```python
from build123d import *

# Parameters (mm, degrees)
BOSS_EXTRUDE1_START       = -4
BOSS_EXTRUDE1_OUTLINE_R   = 2.2
BOSS_EXTRUDE1_OUTLINE_R_2 = 1.025
BOSS_EXTRUDE1_OUTLINE_R_3 = 6.575
BOSS_EXTRUDE1_DEPTH       = 4
SKETCH3_R                 = 8.875
SKETCH3_R_2               = 7.075
CUT_EXTRUDE1_DEPTH        = 1.05
BOSS_EXTRUDE2_START       = -4
SKETCH4_R                 = 1.025
BOSS_EXTRUDE2_DEPTH       = 0.75
FILLET1_R                 = 1
BOSS_EXTRUDE3_START       = -5
SKETCH5_R                 = 32.5
SKETCH5_R_2               = 1.025
SKETCH5_R_3               = 8.875
BOSS_EXTRUDE3_DEPTH       = 5
SKETCH6_R                 = 2.65
CUT_EXTRUDE2_DEPTH        = 5
SKETCH7_R                 = 20.6
SKETCH7_R_2               = 15.6
CUT_EXTRUDE3_DEPTH        = 2.5
BOSS_EXTRUDE4_START       = 1
SKETCH8_R                 = 1.025
BOSS_EXTRUDE4_DEPTH       = 1


# Read off the part's stored shape, not the designer's step: Boss-Extrude1
with BuildPart() as part:
    # Boss-Extrude1 outline → Boss-Extrude1 (new body)
    with BuildSketch(Plane.XY.offset(BOSS_EXTRUDE1_START)):
        with BuildLine():
            Line((-5.8, 12.8), (-5.8, -12.8))
            ThreePointArc((-5.8, -12.8), (-1.992388155, -21.992388155), (7.2, -25.8))
            Line((7.2, -25.8), (32.8, -25.8))
            ThreePointArc((32.8, -25.8), (41.992388155, -21.992388155), (45.8, -12.8))
            Line((45.8, -12.8), (45.8, 12.8))
            ThreePointArc((45.8, 12.8), (41.992388155, 21.992388155), (32.8, 25.8))
            Line((32.8, 25.8), (7.2, 25.8))
            ThreePointArc((7.2, 25.8), (-1.992388155, 21.992388155), (-5.8, 12.8))
        make_face()
        with Locations((25, -22)):
            Circle(BOSS_EXTRUDE1_OUTLINE_R, mode=Mode.SUBTRACT)
        with Locations((20, -11.1252)):
            Circle(BOSS_EXTRUDE1_OUTLINE_R_2, mode=Mode.SUBTRACT)
        with Locations((-2, 0)):
            Circle(BOSS_EXTRUDE1_OUTLINE_R, mode=Mode.SUBTRACT)
        with Locations((20, 0)):
            Circle(BOSS_EXTRUDE1_OUTLINE_R_3, mode=Mode.SUBTRACT)
        with Locations((20, 11.1252)):
            Circle(BOSS_EXTRUDE1_OUTLINE_R_2, mode=Mode.SUBTRACT)
        with Locations((42, 0)):
            Circle(BOSS_EXTRUDE1_OUTLINE_R, mode=Mode.SUBTRACT)
        with Locations((25, 22)):
            Circle(BOSS_EXTRUDE1_OUTLINE_R, mode=Mode.SUBTRACT)
    extrude(amount=BOSS_EXTRUDE1_DEPTH)

    # Sketch3 → Cut-Extrude1 (cut)
    with BuildSketch(Plane.XY):
        with Locations((20, 0)):
            Circle(SKETCH3_R)
        with Locations((20, 0)):
            Circle(SKETCH3_R_2, mode=Mode.SUBTRACT)
    extrude(amount=-CUT_EXTRUDE1_DEPTH, mode=Mode.SUBTRACT)

    # Sketch4 → Boss-Extrude2 (add)
    with BuildSketch(Plane.XY.offset(BOSS_EXTRUDE2_START)):
        with Locations((20, 11.1252)):
            Circle(SKETCH4_R)
        with Locations((20, -11.1252)):
            Circle(SKETCH4_R)
    extrude(amount=BOSS_EXTRUDE2_DEPTH)

    # Fillet1
    fillet1_edges = [part.edges().sort_by_distance(p)[0] for p in [
        (18.975, 11.1252, -3.25),
        (18.975, -11.1252, -3.25),
    ]]
    fillet(fillet1_edges, radius=FILLET1_R)

    # Sketch5 → Boss-Extrude3 (add)
    with BuildSketch(Plane.XY.offset(BOSS_EXTRUDE3_START)):
        with Locations((20, 0)):
            Circle(SKETCH5_R)
        with Locations((20, -11.1252)):
            Circle(SKETCH5_R_2, mode=Mode.SUBTRACT)
        with Locations((20, 11.1252)):
            Circle(SKETCH5_R_2, mode=Mode.SUBTRACT)
        with Locations((20, 0)):
            Circle(SKETCH5_R_3, mode=Mode.SUBTRACT)
    extrude(amount=BOSS_EXTRUDE3_DEPTH)

    # Sketch6 → Cut-Extrude2 (cut)
    with BuildSketch(Plane.XY):
        with Locations((-8.5, 0)):
            Circle(SKETCH6_R)
        with Locations((20, 28.5)):
            Circle(SKETCH6_R)
        with Locations((48.5, 0)):
            Circle(SKETCH6_R)
        with Locations((20, -28.5)):
            Circle(SKETCH6_R)
    extrude(amount=-CUT_EXTRUDE2_DEPTH, mode=Mode.SUBTRACT)

    # Sketch7 → Cut-Extrude3 (cut)
    with BuildSketch(Plane(origin=(0, 0, -5), x_dir=(-1, 0, 0), z_dir=(0, 0, -1))):
        with Locations((-20, 0)):
            Circle(SKETCH7_R)
        with Locations((-20, 0)):
            Circle(SKETCH7_R_2, mode=Mode.SUBTRACT)
    extrude(amount=-CUT_EXTRUDE3_DEPTH, mode=Mode.SUBTRACT)

    # Sketch8 → Boss-Extrude4 (add)
    with BuildSketch(Plane(origin=(0, 0, -4), x_dir=(-1, 0, 0), z_dir=(0, 0, -1)).offset(BOSS_EXTRUDE4_START)):
        with Locations(Location((-20, -11.1252, 0), (0, 0, 180))):
            Circle(SKETCH8_R)
        with Locations(Location((-20, 11.1252, 0), (0, 0, 180))):
            Circle(SKETCH8_R)
    extrude(amount=-BOSS_EXTRUDE4_DEPTH)


solid = part.part
```
Check sheet for the modelled part. Datum: model origin and axes. Units: mm. A direction names the side the tool comes from. Coordinates: 2 decimals unless noted, no trailing zeros. Order: outer loops, then holes, each group sorted by start corner. A loop starts at its lowest first (then second) coordinate and runs counter-clockwise, first axis right, second up. Notation, with made-up numbers: M 9.25,20 L 44.25,20 A32 cw 44.25,58 Z; hole C 41,48.5 d5. An arc over 180 degrees is marked long. Write each question's results on one line, items separated by ' | '. Start each with the question number.
1. Material ranges on probe 1 along Y at (x, z) = (20, -4.35) (3 decimals); probe 2 along Y at (x, z) = (20, -1.85) (3 decimals); probe 3 along X at (y, z) = (-6, -3.9), recorded low to high.
2. Cross-section at A-A on y = 28.5. Record the cut outline in (x, z).
3. Cross-section at C-C on y = 0. State how many separate pieces and enclosed holes the cut face has, and give its area (3 significant figures).
4. Mould release check, pull along X, two halves, no side actions. Record for faces 1 (the face through (36.35, -12.53, -3.77)), 2 (the face through (41, 0, -5)): +X half, -X half, draft (parallel to the pull), parting line (faces both ways), or undercut.
5. Cross-section at B-B on x = 48.5. Record the cut outline in (y, z), and give its area (3 significant figures).
6. Access from +Z, -Z, +X, -X, +Y, -Y to the whole of each face (thin tool, end or side, straight path). Record for faces 3 (the face through (5.12, 4.69, -3.77)), 4 (the face through (18.466, -6.907, -0.518)), 5 (the face through (27, 7, -5)).
7. Cross-section at D-D on x = 10. Record the cut outline in (y, z), and give its area (3 significant figures).
8. Go/stop test with flat-tipped pins: P1, Ø14, axis at x = 20, y = 0, coming from the -Z side; P2, Ø1.5, axis at y = 14.5, z = -1, coming from the -X side; P3, Ø2, axis at y = -11, z = -1, coming from the -X side. Record where each tip stops, or that it passes through.
Checks:
1) probe 1: y = -32.5 to -31.15, -25.85 to -20.6, -15.6 to -8.875, 8.875 to 15.6, 20.6 to 25.85, 31.15 to 32.5 | probe 2: y = -32.5 to -31.15, -25.85 to -12.15, -10.1 to -6.575, 6.575 to 10.1, 12.15 to 25.85, 31.15 to 32.5 | probe 3: x = -11.94 to 0.29, 5.6 to 17.31, 22.69 to 34.4, 39.71 to 51.94
2) outline: M 4.38,-5 L 17.35,-5 L 17.35,0 L 4.38,0 Z; M 22.65,-5 L 35.62,-5 L 35.62,0 L 22.65,0 Z
3) separate pieces: 4 | enclosed holes: 0 | area: 173 mm²
4) face 1: undercut | face 2: draft
5) outline: M -15.62,-5 L -2.65,-5 L -2.65,0 L -15.62,0 Z; M 2.65,-5 L 15.62,-5 L 15.62,0 L 2.65,0 Z | area: 130 mm²
6) face 3: -Z | face 4: +Z | face 5: -Z, +X, -X, +Y, -Y
7) outline: M -30.92,-5 L -18.01,-5 L -18.01,-2.5 L -11.97,-2.5 L -11.97,-5 L 11.97,-5 L 11.97,-2.5 L 18.01,-2.5 L 18.01,-5 L 30.92,-5 L 30.92,0 L -30.92,0 Z | area: 279 mm²
8) P1: stops at z = -4 | P2: stops at x = -9.45 | P3: stops at x = -10.92
